```python
from build123d import *

# Parameters (mm, degrees)
SKETCH1_R               = 1.5
BOSS_EXTRUDE1_DEPTH     = 105
FILLET1_R               = 10
CUT_EXTRUDE1_DEPTH      = 117.542660484
CUT_EXTRUDE1_DEPTH_BACK = 117.542660484
CAVITY1_DEPTH           = 3
SKETCH3_R               = 2.5
SKETCH3_R_2             = 1.5
BOSS_EXTRUDE2_DEPTH     = 20
BOSS_EXTRUDE3_REACH     = 134.065
SKETCH4_R               = 1.5
CUT_EXTRUDE2_DEPTH      = 135.841357497
CUT_EXTRUDE2_DEPTH_BACK = 135.841357497
FILLET2_R               = 5
CUT_EXTRUDE3_DEPTH      = 10


# Read off the part's stored shape, not the designer's step: Cavity1
with BuildPart() as part:
    # Sketch1 → Boss-Extrude1 (new body)
    with BuildSketch(Plane(origin=(0, 0, 0), x_dir=(0, 0, -1), z_dir=(1, 0, 0))):
        with BuildLine():
            add(Edge.make_bspline(
                [(3.73e-07, 7.5), (-15, 0), (-3.73e-07, -7.5)],
                knots=[0, 0, 0, 1, 1, 1], degree=2, weights=[1, 2.333333333, 1]))
            add(Edge.make_bspline(
                [(3.73e-07, 7.5), (100, 0), (-3.73e-07, -7.5)],
                knots=[0, 0, 0, 1, 1, 1], degree=2, weights=[1, 1.001467765, 1]))
        make_face()
        Circle(SKETCH1_R, mode=Mode.SUBTRACT)
    extrude(amount=BOSS_EXTRUDE1_DEPTH)

    # Fillet1
    fillet1_edges = [part.edges().sort_by_distance(p)[0] for p in [
        (52.5, -7.5, 3.73e-07),
        (52.5, 7.5, -3.73e-07),
    ]]
    fillet(fillet1_edges, radius=FILLET1_R)

    # Sketch2 → Cut-Extrude1 (cut, two sides: drawn at the far end of the back side and taken through both)
    with BuildSketch(Plane(origin=(0, 0, 0), x_dir=(1, 0, 0), z_dir=(0, 1, 0)).offset(-CUT_EXTRUDE1_DEPTH_BACK)):
        with BuildLine():
            Line((65, 19.76833361), (65, 24.578179161))
            ThreePointArc((65, 24.578179161), (52.5, 34.902500415), (40, 24.578179161))
            Line((40, 24.578179161), (40, 19.76833361))
            Line((40, 19.76833361), (40, 14.958488059))
            ThreePointArc((40, 14.958488059), (52.5, 4.634166805), (65, 14.958488059))
            Line((65, 14.958488059), (65, 19.76833361))
        make_face()
        with BuildLine():
            Line((65, 24.578179161), (65, 50.03666722))
            Line((65, 50.03666722), (40, 50.03666722))
            Line((40, 50.03666722), (40, 24.578179161))
            ThreePointArc((40, 24.578179161), (52.5, 34.902500415), (65, 24.578179161))
        make_face()
    extrude(amount=CUT_EXTRUDE1_DEPTH + CUT_EXTRUDE1_DEPTH_BACK, mode=Mode.SUBTRACT)

    # Cavity1 outline → Cavity1 (cut)
    with BuildSketch(Plane.YZ):
        with BuildLine():
            ThreePointArc((-2, -13.75), (0, -15.75), (2, -13.75))
            Line((2, -13.75), (2.497863905, -2.796994085))
            ThreePointArc((2.497863905, -2.796994085), (0, 3.75), (-2.497863905, -2.796994085))
            Line((-2.497863905, -2.796994085), (-2, -13.75))
        make_face()
    extrude(amount=CAVITY1_DEPTH, mode=Mode.SUBTRACT)

    # Sketch3 → Boss-Extrude2 (add)
    # profile 1 of 2: a face of its own
    with BuildSketch(Plane(origin=(105, 0, 0), x_dir=(0, 0, -1), z_dir=(1, 0, 0))):
        Circle(SKETCH3_R)
        with Locations(Location((0, 0, 0), (0, 0, 180))):
            Circle(SKETCH3_R_2, mode=Mode.SUBTRACT)
    # profile 2 of 2: a face of its own
    with BuildSketch(Plane(origin=(105, 0, 0), x_dir=(0, 0, -1), z_dir=(1, 0, 0))):
        with Locations(Location((0, 0, 0), (0, 0, 180))):
            Circle(SKETCH3_R_2)
    extrude(amount=BOSS_EXTRUDE2_DEPTH)

    # Sketch4 → Boss-Extrude3 (add, up to next)
    with BuildSketch(Plane.ZY.offset(-3), mode=Mode.PRIVATE) as boss_extrude3_sk1:
        Circle(SKETCH4_R)
    boss_extrude3_tool1 = extrude(boss_extrude3_sk1.sketch, amount=-BOSS_EXTRUDE3_REACH, mode=Mode.PRIVATE) - part.part
    add(boss_extrude3_tool1.solids().sort_by_distance((3, 0, 0))[0])

    # Sketch5 → Cut-Extrude2 (cut, two sides: drawn at the far end of the back side and taken through both)
    with BuildSketch(Plane(origin=(0, 0, 0), x_dir=(1, 0, 0), z_dir=(0, 1, 0)).offset(-CUT_EXTRUDE2_DEPTH_BACK)):
        Polygon((40, 14.958488059), (35, 50.03666722), (40, 50.03666722), align=None)
        Polygon((65, 50.03666722), (70, 50.03666722), (65, 14.958488059), align=None)
    extrude(amount=CUT_EXTRUDE2_DEPTH + CUT_EXTRUDE2_DEPTH_BACK, mode=Mode.SUBTRACT)

    # Fillet2
    fillet2_edges = [part.edges().sort_by_distance(p)[0] for p in [
        (1.5, 2.497863905, -2.796994085),
        (1.5, -2.497863905, -2.796994085),
    ]]
    fillet(fillet2_edges, radius=FILLET2_R)

    # Sketch7 → Cut-Extrude3 (cut)
    with BuildSketch(Plane.ZY.offset(-3)):
        with BuildLine():
            Line((-13.754651281, -2.199995083), (-4.420599378, -2.62427017))
            ThreePointArc((-4.420599378, -2.62427017), (-3.210509972, -2.836668826), (-2.093976777, -3.349292651))
            ThreePointArc((-2.093976777, -3.349292651), (3.95, 0), (-2.093976777, 3.349292651))
            ThreePointArc((-2.093976777, 3.349292651), (-3.210509972, 2.836668826), (-4.420599378, 2.62427017))
            Line((-4.420599378, 2.62427017), (-13.754651281, 2.199995083))
            ThreePointArc((-13.754651281, 2.199995083), (-15.95, 0), (-13.754651281, -2.199995083))
        make_face()
        with BuildLine():
            Line((-4.411517846, 2.424476462), (-13.75, 2))
            ThreePointArc((-13.75, 2), (-15.75, 0), (-13.75, -2))
            Line((-13.75, -2), (-4.411517846, -2.424476462))
            ThreePointArc((-4.411517846, -2.424476462), (-3.151008047, -2.645725062), (-1.987952636, -3.179708213))
            ThreePointArc((-1.987952636, -3.179708213), (3.75, 0), (-1.987952636, 3.179708213))
            ThreePointArc((-1.987952636, 3.179708213), (-3.151008047, 2.645725062), (-4.411517846, 2.424476462))
        make_face(mode=Mode.SUBTRACT)
    extrude(amount=CUT_EXTRUDE3_DEPTH, mode=Mode.SUBTRACT)


solid = part.part
```
CAD build for the part. Positions are in the model's coordinates, mm. A direction names the side the tool comes from. Give positions to 0.01 mm unless a question says otherwise; leave off trailing zeros. Order: outer loops, then holes, each group sorted by start corner. A loop starts at its lowest first (then second) coordinate and runs counter-clockwise, first axis right, second up. Notation, with made-up numbers: M 52.5,82.25 L 76.5,82.25 A21 cw 76.5,107.25 Z; hole C 16,17 d7. An arc over 180 degrees is marked long. Put each result on its own line as item: value. Start each with the question number.
(1) Mould opens along X. For faces 1 (the flat face through (3, 0, -6)), 2 (the flat face through (38.09, -0.09, -28.35)), 3 (the flat face through (1.521, 2.415, -9.022)) say: +X half, -X half, draft (parallel to the pull), parting line (faces both ways), or undercut.
(2) Saw through at A-A, the plane x = 111. Write the cut outline in (y, z), then the cut area to 3 significant figures.
(3) Which spindle directions (+Z, -Z, +X, -X, +Y, -Y) get a long thin tool onto all of the face, cutting with end or side? Do faces 4 (the cylindrical face through (114.86, -2.44, 0.54)), 5 (the cylindrical face through (1.521, 2.842, -3.194)), 6 (the flat face through (67, 0, -29)). Say none if no direction does.
(4) Flat gauge pins, fed straight in: pin 1 Ø2 at (x, z) = (43.5, 4) entering from -Y; pin 2 Ø1 at (x, y) = (101.5, -2.5) entering from +Z; pin 3 Ø1.5 at (x, y) = (46, 2) entering from +Z. Where does each tip first touch, or does it go through?
(5) Drill centre lines: line 1 along Z through (x, y) = (1, 0); line 2 along X through (y, z) = (-6, 0.5); line 3 along Y through (x, z) = (1.15, 0). Where is each one in solid material? Low to high.
Check result:
1. face 1: -X half
1. face 2: undercut
1. face 3: draft
2. outline: C 0,0 d5
2. area: 19.6 mm2
3. face 4: +X
3. face 5: -X
3. face 6: -Z, +Y, -Y
4. pin 1: stops at y = -5.97
4. pin 2: stops at z = 9.34
4. pin 3: stops at z = 10.03
5. line 1: z = -50.04 to -15.95, 3.95 to 10.5
5. line 2: x = 0 to 105
5. line 3: y = -7.11 to -3.95, 3.95 to 7.11
